Verification items for the finished model (mm, model axes). A direction names the side the tool comes from. Coordinates: 2 decimals unless noted, no trailing zeros. Write each loop counter-clockwise with the first axis right and the second up, starting at its lowest first coordinate (ties: lowest second). Pieces come first, ordered by that corner, then holes. Notation, with made-up numbers: M 50,46 L 69,46 A12 cw 69,68 Z; hole C 27.5,2 d7. An arc over 180 degrees is marked long. One line per item, written item: value.
```python
from build123d import *

# Parameters (mm, degrees)
PAD_DEPTH       = 5.5
SKETCH006_R     = 2
POCKET001_DEPTH = 50
SKETCH004_R     = 5.5
POCKET_DEPTH    = 3.5
PAD001_DEPTH    = 6
FILLET_R        = 3


with BuildPart() as pocket:
    # Sketch → Pad (new body)
    with BuildSketch(Plane.XY.offset(6)):
        with BuildLine():
            ThreePointArc((6.65, 0), (0, 6.65), (-6.65, 0))
            Line((-6.65, 0), (-6.65, -9))
            Line((-6.65, -9), (-25.186368, -9))
            Line((-25.186368, -9), (-25.186368, 9))
            Line((-25.186368, 9), (29.813632, 9))
            Line((29.813632, 9), (29.813632, -9))
            Line((29.813632, -9), (6.65, -9))
            Line((6.65, 0), (6.65, -9))
        make_face()
    extrude(amount=PAD_DEPTH)

    # Sketch006 → Pocket001 (cut)
    with BuildSketch(Plane(origin=(0, -9, 6), x_dir=(1, 0, 0), z_dir=(0, -1, 0))):
        with Locations((-22.194616, 2.739605)):
            Circle(SKETCH006_R)
    extrude(amount=-POCKET001_DEPTH, mode=Mode.SUBTRACT)

    # Sketch004 → Pocket (cut)
    with BuildSketch(Plane.XY.offset(11.5)):
        with Locations((15.55286, 0)):
            Circle(SKETCH004_R)
    extrude(amount=-POCKET_DEPTH, mode=Mode.SUBTRACT)


with BuildPart() as fillet_body:
    # Sketch005 → Pad001 (new body)
    with BuildSketch(Plane(origin=(0, 0, 0), x_dir=(1, 0, 0), z_dir=(0, 0, -1))):
        with BuildLine():
            ThreePointArc((-8.5, 0), (0, -8.5), (8.5, 0))
            Line((8.5, 0), (8.5, 9))
            Line((8.5, 9), (11.167023, 9))
            ThreePointArc((11.167023, -9), (14.342329, 0), (11.167023, 9))
            Line((-12.044614, -9), (11.167023, -9))
            ThreePointArc((-11.167023, 9), (-14.785971, 0.155049), (-12.044614, -9))
            Line((-8.5, 9), (-11.167023, 9))
            Line((-8.5, 0), (-8.5, 9))
        make_face()
    extrude(amount=-PAD001_DEPTH)

    # Fusion: union Pocket
    add(pocket.part)

    # Fillet
    fillet_edges = [fillet_body.edges().sort_by_distance(p)[0] for p in [
        (-25.186368, 0, 6),
        (29.813632, 0, 6),
    ]]
    fillet(fillet_edges, radius=FILLET_R)


solid = fillet_body.part
```
Item 1: Access from +Z, -Z, +X, -X, +Y, -Y to the whole of each face (thin tool, end or side, straight path). Record for faces 1 (the face through (20.63, -2.11, 9.77)), 2 (the face through (-14.78, -0.29, 2.96)), 3 (the face through (-8.5, -4, 3)), 4 (the face through (14.34, 0.14, 2.96)).
The answers:
face 1: +Z
face 2: -Z, -X
face 3: -Z, -Y
face 4: -Z, +X
Item 2: Draft check along X on faces 5 (the face through (-18, 0, 6)), 6 (the face through (-25.186, 0, 10)), 7 (the face through (6.65, -4, 9)), 8 (the face through (29.814, 0, 10)). Enter one of: released by +X, released by -X, zero draft, split by the parting line, or undercut.
The answers:
face 5: zero draft
face 6: released by -X
face 7: undercut
face 8: released by +X
Item 3: Cross-section at B-B, the plane z = 10. Enter the section's corners in (x, y), and give its area (3 significant figures).
The answers:
outline: M -25.19,-9 L -23.75,-9 L -23.75,9 L -25.19,9 Z; M -20.64,-9 L -6.65,-9 L -6.65,0 A6.65 cw 6.65,0 L 6.65,-9 L 29.81,-9 L 29.81,9 L -20.64,9 Z; hole C 15.55,0 d11
area: 650 mm²
Item 4: Cross-section at D-D, the plane x = -19. Enter the section's corners in (y, z).
The answers:
outline: M -9,6 L 9,6 L 9,11.5 L -9,11.5 Z
Item 5: Cross-section at A-A, the plane y = 1.25. Enter the section's corners in (x, z), and give its area (3 significant figures).
The answers:
outline: M -25.19,9 A3 ccw -22.19,6 L -14.79,6 L -14.79,0 L -8.41,0 L -8.41,6 L -6.53,6 L -6.53,11.5 L -25.19,11.5 Z; M 6.53,6 L 8.41,6 L 8.41,0 L 14.29,0 L 14.29,6 L 26.81,6 A3 ccw 29.81,9 L 29.81,11.5 L 20.91,11.5 L 20.91,8 L 10.2,8 L 10.2,11.5 L 6.53,11.5 Z; hole C -22.19,8.74 d4
area: 250 mm²
Item 6: Go/stop test with flat-tipped pins: P1, Ø5, axis at y = -6.5, z = 2.5, coming from the -X side; P2, Ø1.5, axis at y = -3.5, z = 3.5, coming from the +X side; P3, Ø8, axis at x = 22.5, y = 0.5, coming from the -Z side. Record where each tip stops, or that it passes through.
The answers:
P1: stops at x = -14.06
P2: stops at x = 14.08
P3: stops at z = 6
Item 7: Cross-section at C-C, the plane x = 0. Enter the section's corners in (y, z).
The answers:
outline: M 6.65,6 L 8.5,6 L 8.5,0 L 9,0 L 9,11.5 L 6.65,11.5 Z
Item 8: Scan lines: line 1 (X direction, y = -2.75, z = 9.25); line 2 (X direction, y = 1, z = 7.5); line 3 (X direction, y = -3.25, z = 8.25). Record each from-to range of solid material in increasing order.
The answers:
line 1: x = -25.19 to -24.13, -20.26 to -6.65, 6.65 to 10.79, 20.32 to 29.81
line 2: x = -24.78 to -23.76, -20.63 to -6.57, 6.57 to 29.41
line 3: x = -25.09 to -24.13, -20.26 to -6.65, 6.65 to 11.12, 19.99 to 29.72
